Geometry check sheet. Reference: the model listing, model coordinates, mm. A direction names the side the tool comes from. Round coordinates to 2 decimals unless told otherwise and drop trailing zeros. Order: outer loops, then holes, each group sorted by start corner. A loop starts at its lowest first (then second) coordinate and runs counter-clockwise, first axis right, second up. Notation, with made-up numbers: (-37.5, 54.5) - (18.5, 54.5) arc R23 cw to (18.5, 90.5) - close; hole circle Ø4 at (76.5, 11.25). An arc over 180 degrees is marked (long way). Answer as CSV lines item,"result". Start each with the question number.
```python
from build123d import *

# Parameters (mm, degrees)
BOSS_EXTRUDE1_DEPTH     = 2.5
SKETCH2_R               = 9.5
BOSS_EXTRUDE2_DEPTH     = 12.5
CUT_EXTRUDE1_DEPTH      = 21.72890494
CUT_EXTRUDE1_DEPTH_BACK = 21.72890494
SKETCH3_R               = 8
FILLET1_R               = 1


with BuildPart() as part:
    # Sketch1 → Boss-Extrude1 (new, symmetric)
    with BuildSketch(Plane.XY):
        Polygon((-12.5, 0), (-6.25, 10.825317547), (6.25, 10.825317547), (12.5, 0), (6.25, -10.825317547), (-6.25, -10.825317547), align=None)
    extrude(amount=BOSS_EXTRUDE1_DEPTH, both=True)

    # Sketch2 → Boss-Extrude2 (add, symmetric)
    with BuildSketch(Plane.XY):
        Circle(SKETCH2_R)
    extrude(amount=BOSS_EXTRUDE2_DEPTH, both=True)

    # Sketch3 → Cut-Extrude1 (cut, two sides: drawn at the far end of the back side and taken through both)
    with BuildSketch(Plane.XY.offset(-CUT_EXTRUDE1_DEPTH_BACK)):
        Circle(SKETCH3_R)
    extrude(amount=CUT_EXTRUDE1_DEPTH + CUT_EXTRUDE1_DEPTH_BACK, mode=Mode.SUBTRACT)

    # Fillet1
    fillet1_edges = [part.edges().sort_by_distance(p)[0] for p in [
        (-9.5, 0, -2.5),
        (-9.5, 0, 2.5),
    ]]
    fillet(fillet1_edges, radius=FILLET1_R)


solid = part.part
```
1. Access from +Z, -Z, +X, -X, +Y, -Y to the whole of each face (thin tool, end or side, straight path). Record for faces 4 (the face through (-9.419, 5.337, 0.035)), 5 (the face through (-10, 4, -2.5)), 6 (the face through (-10, 4, 2.5)).
2. Section check B-B on z = 4.5. Record the boundary of the cut face in (x, y).
3. Draft check along X on faces 1 (the face through (-4.3, -7, -12.5)), 2 (the face through (-1.73, -7.81, -0.18)), 3 (the face through (9.419, -5.337, 0.035)). Enter one of: released by +X, released by -X, zero draft, split by the parting line, or undercut.
4. Section check A-A on x = 0. Record the boundary of the cut face in (y, z).
5. Thickness scan on probe 1 along Y at (x, z) = (-0.25, 9.5); probe 2 along Y at (x, z) = (0, 2.25); probe 3 along X at (y, z) = (-2.25, 7.25). Record the ranges inside material, lowest first.
6. Go/stop test with flat-tipped pins: pin 1 Ø1 at (x, z) = (2.5, -4.5) entering from +Y; pin 2 Ø6 at (x, z) = (-9.5, -5.5) entering from +Y; pin 3 Ø6 at (y, z) = (-6, -9.5) entering from +X; pin 4 Ø1.5 at (x, y) = (2, -7.5) entering from -Z. Record where each tip stops, or that it passes through.
Numbers:
1,face 4,"+Z, -Z, -X, +Y"
1,face 5,"-Z"
1,face 6,"+Z"
2,outline,"circle Ø19 at (0, 0); hole circle Ø16 at (0, 0)"
3,face 1,"zero draft"
3,face 2,"undercut"
3,face 3,"released by +X"
4,outline,"(-10.83, -2.5) - (-10.5, -2.5) arc R1 cw to (-9.5, -3.5) - (-9.5, -12.5) - (-8, -12.5) - (-8, 12.5) - (-9.5, 12.5) - (-9.5, 3.5) arc R1 cw to (-10.5, 2.5) - (-10.83, 2.5) - close; (8, -12.5) - (9.5, -12.5) - (9.5, -3.5) arc R1 cw to (10.5, -2.5) - (10.83, -2.5) - (10.83, 2.5) - (10.5, 2.5) arc R1 cw to (9.5, 3.5) - (9.5, 12.5) - (8, 12.5) - close"
5,probe 1,"y = -9.5 to -8, 8 to 9.5"
5,probe 2,"y = -10.83 to -8, 8 to 10.83"
5,probe 3,"x = -9.23 to -7.68, 7.68 to 9.23"
6,pin 1,"stops at y = 9.29"
6,pin 2,"stops at y = 6.93"
6,pin 3,"stops at x = 9.01"
6,pin 4,"stops at z = -12.5"
